CAD build for the part. Positions are in the model's coordinates, mm. Face numbers are marked on the shaded views. A direction names the side the tool comes from. Coordinates: 2 decimals unless noted, no trailing zeros. Order: outer loops, then holes, each group sorted by start corner. A loop starts at its lowest first (then second) coordinate and runs counter-clockwise, first axis right, second up. Notation, with made-up numbers: (-25, -0.75) -> (-18, -0.75) arc R31 cw to (-18, 36.25) -> close; hole circle Ø8 at (41.25, 39). An arc over 180 degrees is marked (long way). Use one line per item in the form item = value. Start each with the question number.
from build123d import *

# Parameters (mm, degrees)
SKETCH_1_W          = 70
SKETCH_1_H          = 40
SKETCH_1_R          = 2.5
EXTRUDE_1_DEPTH     = 5
EXTRUDE_2_DEPTH     = 60
CUT_EXTRUDE_1_DEPTH = 100
EXTRUDE_3_DEPTH     = 30
CUT_EXTRUDE_2_DEPTH = 70
SKETCH_8_R          = 6
SKETCH_8_R_2        = 0.75
CUT_EXTRUDE_3_DEPTH = 5


with BuildPart() as part:
    # 草图1 → 凸台-拉伸1 (new body)
    with BuildSketch(Plane.XY):
        Rectangle(SKETCH_1_W, SKETCH_1_H)
        with Locations((-20, 10)):
            Circle(SKETCH_1_R, mode=Mode.SUBTRACT)
        with Locations((20, 10)):
            Circle(SKETCH_1_R, mode=Mode.SUBTRACT)
        with Locations((-20, -10)):
            Circle(SKETCH_1_R, mode=Mode.SUBTRACT)
        with Locations((20, -10)):
            Circle(SKETCH_1_R, mode=Mode.SUBTRACT)
    extrude(amount=EXTRUDE_1_DEPTH)

    # 草图3 → 凸台-拉伸2 (add)
    with BuildSketch(Plane.XY.offset(5)):
        Polygon((-35, -20), (35, -20), (35, 20), (30, 20), (30, -15), (-30, -15), (-30, 20), (-35, 20), align=None)
    extrude(amount=EXTRUDE_2_DEPTH)

    # 草图4 → 切除-拉伸1 (cut)
    with BuildSketch(Plane.ZY.offset(35)):
        Polygon((5, 20), (65, -15), (65, 20), align=None)
    extrude(amount=-CUT_EXTRUDE_1_DEPTH, mode=Mode.SUBTRACT)

    # 草图5 → 凸台-拉伸3 (add)
    with BuildSketch(Plane.XZ.offset(20)):
        Polygon((30, 0), (35, 0), (35, 65), (-35, 65), (-35, 0), (-30, 0), (-30, 62), (30, 62), align=None)
    extrude(amount=EXTRUDE_3_DEPTH)

    # 草图6 → 切除-拉伸2 (cut)
    with BuildSketch(Plane.ZY.offset(35)):
        Polygon((62, -50), (0, -20), (0, -50), align=None)
    extrude(amount=-CUT_EXTRUDE_2_DEPTH, mode=Mode.SUBTRACT)

    # 草图8 → 切除-拉伸3 (cut)
    with BuildSketch(Plane.XY.offset(65)):
        with Locations((-10, -35)):
            Circle(SKETCH_8_R)
        with Locations((18, -35)):
            Circle(SKETCH_8_R_2)
        with Locations((11, -43)):
            Circle(SKETCH_8_R_2)
        with Locations((0, -44)):
            Circle(SKETCH_8_R_2)
        with Locations((11, -27)):
            Circle(SKETCH_8_R_2)
        with Locations((0, -26)):
            Circle(SKETCH_8_R_2)
    extrude(amount=-CUT_EXTRUDE_3_DEPTH, mode=Mode.SUBTRACT)


solid = part.part
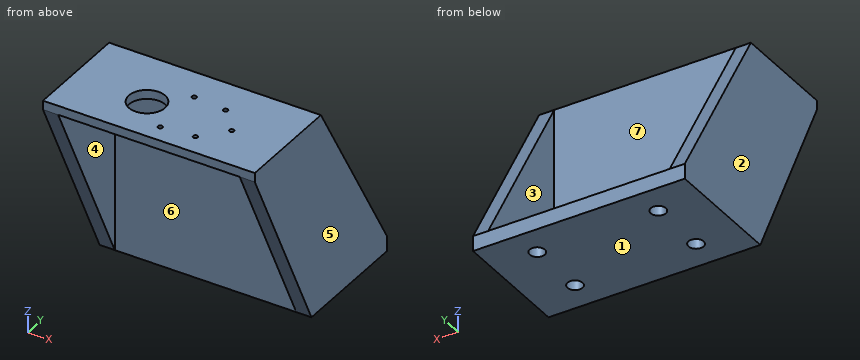
1) Drop flat-ended pins along their axis: P1, Ø10, axis at x = 18, z = 45, coming from the +Y side; P2, Ø1.7, axis at x = 0, y = -26, coming from the +Z side; P3, Ø2, axis at x = 0, y = -44, coming from the -Z side; P4, Ø8, axis at x = 19, z = 41, coming from the -Y side. Give the stop position or say it passes through.
2) Cut at B-B on y = -31.5. Give the cut face in (x, z), then the cut area to 3 significant figures.
3) Two-plate mould, pull along X, no slides. Class the marked faces 1, 2, 3 and 4: released by +X, released by -X, zero draft, split by the parting line, or undercut.
4) Probe L1, parallel to Y at x = 11, z = 63.3; L2, parallel to Y at x = 20, z = 3; L3, parallel to X at y = -21.5, z = 26.5. List the from-to ranges inside material, lowest first.
5) 3-axis set-ups, long thin cutter, end or side, ignore diameter. For the marked faces 5, 6 and 7: which of +Z, -Z, +X, -X, +Y, -Y reach the whole face in a straight line?
6) Cut at C-C on z = 51.5. Give the cut face in (x, y) (3 decimals), then the cut area to 3 significant figures.
7) Cut at D-D on y = -2. Give the cut face in (x, z), then the cut area to 3 significant figures.
8) Cut at A-A on x = -10. Give the cut face in (y, z), then the cut area to 3 significant figures.
Values follow:
q1.P1 = -15
q1.P2 = 65
q1.P3 = 62
q1.P4 = -20
q2.outline = (-35, 23.77) -> (-30, 23.77) -> (-30, 62) -> (-14.87, 62) -> (-14.87, 65) -> (-35, 65) -> close; (-5.13, 62) -> (30, 62) -> (30, 23.77) -> (35, 23.77) -> (35, 65) -> (-5.13, 65) -> close
q2.area = 563 mm^2
q3.face_1 = zero draft
q3.face_2 = released by -X
q3.face_3 = undercut
q3.face_4 = undercut
q4.L1 = -50 to -43.75, -42.25 to -27.75, -26.25 to -15
q4.L2 = -20 to -12.5, -7.5 to 7.5, 12.5 to 20
q4.L3 = -35 to -30, 30 to 35
q5.face_5 = +Z, -Z, +X, +Y, -Y
q5.face_6 = -Z, -Y
q5.face_7 = +Z, +Y
q6.outline = (-35, -44.919) -> (-30, -44.919) -> (-30, -20) -> (30, -20) -> (30, -44.919) -> (35, -44.919) -> (35, -7.125) -> (30, -7.125) -> (30, -15) -> (-30, -15) -> (-30, -7.125) -> (-35, -7.125) -> close
q6.area = 678 mm^2
q7.outline = (-35, 0) -> (35, 0) -> (35, 42.71) -> (30, 42.71) -> (30, 5) -> (-30, 5) -> (-30, 42.71) -> (-35, 42.71) -> close
q7.area = 727 mm^2
q8.outline = (-50, 62) -> (-41, 62) -> (-41, 65) -> (-50, 65) -> close; (-29, 62) -> (-20, 62) -> (-20, 0) -> (20, 0) -> (20, 5) -> (-15, 5) -> (-15, 65) -> (-29, 65) -> close
q8.area = 554 mm^2
